```python
from build123d import *

# Parameters (mm, degrees)
F0_W     = 355.6
F0_H     = 50.8
F0_R     = 6.35
F1_DEPTH = 5.334
F2_R     = 2.54
F4_DEPTH = 25.4


with BuildPart() as f1:
    # F0 (on Right) → F1 (new body)
    with BuildSketch(Plane.YZ):
        with Locations((-62.0332211256, -100.6222862377)):
            Rectangle(F0_W, F0_H)
        with Locations((-213.1684422493, -100.6222862377)):
            Circle(F0_R, mode=Mode.SUBTRACT)
        with Locations((90.3667788744, -100.6222862377)):
            Circle(F0_R, mode=Mode.SUBTRACT)
    extrude(amount=F1_DEPTH)

    # F2
    f2_edges = [f1.edges().sort_by_distance(p)[0] for p in [
        (2.667, 115.766779, -126.022286),
        (2.667, 115.766779, -75.222286),
        (2.667, -239.833221, -75.222286),
    ]]
    fillet(f2_edges, radius=F2_R)

    # F3 (on face) → F4 (cut)
    with BuildSketch(Plane.YZ.offset(5.334)):
        with BuildLine():
            ThreePointArc((-204.111539145, -78.5993967268), (-201.2621922493, -80.0000563101), (-198.6245120203, -81.7673333143))
            ThreePointArc((-198.6245120203, -81.7673333143), (-198.2244908381, -80.9236336682), (-198.0871922493, -80.0000563101))
            ThreePointArc((-198.0871922493, -80.0000563101), (-200.5431829982, -76.9075410398), (-204.111539145, -78.5993967268))
        make_face()
        with BuildLine():
            ThreePointArc((-227.7123724783, -81.7673333143), (-225.0746922493, -80.0000563101), (-222.2253453536, -78.5993967268))
            ThreePointArc((-222.2253453536, -78.5993967268), (-226.6621922493, -77.2504256531), (-227.7123724783, -81.7673333143))
        make_face()
        with BuildLine():
            ThreePointArc((-221.8996922493, -80.0000563101), (-221.982176979, -79.281047059), (-222.2253453536, -78.5993967268))
            ThreePointArc((-222.2253453536, -78.5993967268), (-225.0746922493, -80.0000563101), (-227.7123724783, -81.7673333143))
            ThreePointArc((-227.7123724783, -81.7673333143), (-224.1511148912, -83.0377577213), (-221.8996922493, -80.0000563101))
        make_face()
        with BuildLine():
            ThreePointArc((-204.111539145, -78.5993967268), (-202.8496922493, -82.7496869671), (-198.6245120203, -81.7673333143))
            ThreePointArc((-198.6245120203, -81.7673333143), (-201.2621922493, -80.0000563101), (-204.111539145, -78.5993967268))
        make_face()
        with BuildLine():
            ThreePointArc((-189.567608916, -103.7902228252), (-189.4089178433, -102.2097862377), (-189.3559422493, -100.6222862377))
            ThreePointArc((-189.3559422493, -100.6222862377), (-189.4089178433, -99.0347862377), (-189.567608916, -97.4543496502))
            ThreePointArc((-189.567608916, -97.4543496502), (-192.5309422493, -100.6222862377), (-189.567608916, -103.7902228252))
        make_face()
        with BuildLine():
            ThreePointArc((-189.567608916, -97.4543496502), (-189.4089178433, -99.0347862377), (-189.3559422493, -100.6222862377))
            ThreePointArc((-189.3559422493, -100.6222862377), (-189.4089178433, -102.2097862377), (-189.567608916, -103.7902228252))
            ThreePointArc((-189.567608916, -103.7902228252), (-187.1870043372, -102.9409783978), (-186.1809422493, -100.6222862377))
            ThreePointArc((-186.1809422493, -100.6222862377), (-187.1870043372, -98.3035940776), (-189.567608916, -97.4543496502))
        make_face()
        with BuildLine():
            ThreePointArc((-198.0871922493, -121.2445161653), (-198.2244908381, -120.3209388072), (-198.6245120203, -119.4772391611))
            ThreePointArc((-198.6245120203, -119.4772391611), (-201.2621922493, -121.2445161653), (-204.111539145, -122.6451757486))
            ThreePointArc((-204.111539145, -122.6451757486), (-200.5431829982, -124.3370314356), (-198.0871922493, -121.2445161653))
        make_face()
        with BuildLine():
            ThreePointArc((-204.111539145, -122.6451757486), (-201.2621922493, -121.2445161653), (-198.6245120203, -119.4772391611))
            ThreePointArc((-198.6245120203, -119.4772391611), (-202.8496922493, -118.4948855083), (-204.111539145, -122.6451757486))
        make_face()
        with BuildLine():
            ThreePointArc((-227.7123724783, -119.4772391611), (-226.6621922493, -123.9941468223), (-222.2253453536, -122.6451757486))
            ThreePointArc((-222.2253453536, -122.6451757486), (-225.0746922493, -121.2445161653), (-227.7123724783, -119.4772391611))
        make_face()
        with BuildLine():
            ThreePointArc((-227.7123724783, -119.4772391611), (-225.0746922493, -121.2445161653), (-222.2253453536, -122.6451757486))
            ThreePointArc((-222.2253453536, -122.6451757486), (-221.982176979, -121.9635254164), (-221.8996922493, -121.2445161653))
            ThreePointArc((-221.8996922493, -121.2445161653), (-224.1511148912, -118.2068147541), (-227.7123724783, -119.4772391611))
        make_face()
    extrude(amount=-F4_DEPTH, mode=Mode.SUBTRACT)


solid = f1.part
```
Check sheet for the modelled part. Datum: model origin and axes. Units: mm. Give positions to 0.01 mm unless a question says otherwise; leave off trailing zeros. Write each loop counter-clockwise with the first axis right and the second up, starting at its lowest first coordinate (ties: lowest second). Pieces come first, ordered by that corner, then holes. Notation, with made-up numbers: (76.25, -40) - (132.25, -40) arc R30 ccw to (132.25, -4) - close; hole circle Ø10 at (52.25, 27). An arc over 180 degrees is marked (long way). Answer as a JSON object with one key per item and string values. Group by question number.
1) Sectioned sample at A-A (x = 4.3). Record the cut outline in (y, z) (3 decimals).
2) Thickness scan on probe 1 along Y at (x, z) = (2.9, -118.5); probe 2 along Y at (x, z) = (4.3, -104); probe 3 along Z at (x, y) = (4.9, -213). Record the ranges inside material, lowest first. Write a range as from..to.
3) Release check for a two-part mould opening along Z. For faces 1 (the face through (5.334, -65, -100)), 2 (the face through (2.63, 85.33, -104.49)) record: pulls with the +Z half, pulls with the -Z half, needs draft (parallel to the pull), parting line crosses it, or undercut.
Geometry results:
{
 "1": {"outline": "(-239.833, -126.022) - (113.227, -126.022) arc R2.54 ccw to (115.767, -123.482) - (115.767, -77.762) arc R2.54 ccw to (113.227, -75.222) - (-237.293, -75.222) arc R2.54 ccw to (-239.833, -77.762) - close; hole circle Ø6.35 at (-225.075, -121.245); hole circle Ø6.35 at (-225.075, -80); hole circle Ø12.7 at (-213.168, -100.622); hole circle Ø6.35 at (-201.262, -121.245); hole circle Ø6.35 at (-201.262, -80); hole circle Ø6.35 at (-189.356, -100.622); hole circle Ø12.7 at (90.367, -100.622)"},
 "2": {"probe 1": "y = -239.83..-226.67, -223.48..-202.86, -199.67..115.77", "probe 2": "y = -239.83..-218.55, -207.79..84.99, 95.74..115.77", "probe 3": "z = -126.02..-106.97, -94.27..-75.22"},
 "3": {"face 1": "needs draft", "face 2": "undercut"}
}
